```python
from build123d import *

# Parameters (mm, degrees)
BOSS_EXTRUDE1_START = -19300
BOSS_EXTRUDE1_DEPTH = 450


with BuildPart() as part:
    # Sketch1 → Boss-Extrude1 (new body)
    with BuildSketch(Plane(origin=(0, 0, 0), x_dir=(1, 0, 0), z_dir=(0, 1, 0)).offset(BOSS_EXTRUDE1_START)):
        Polygon((175, 300), (-175, 300), (-275, 200), (-200, -300), (-25, -300), (-25, -200), (25, -200), (25, -300), (200, -300), (275, 200), align=None)
    extrude(amount=BOSS_EXTRUDE1_DEPTH)


solid = part.part
```
Build history of the part. All positions in model axes, mm. A direction names the side the tool comes from. Give positions to 0.01 mm unless a question says otherwise; leave off trailing zeros. Loops run counter-clockwise (first coordinate to the right, second up) from the corner with the lowest first, then second, coordinate; pieces in that order, holes last.
1) 3-axis set-ups, long thin cutter, end or side, ignore diameter. For faces 1 (the face through (25, -19078, 249)), 2 (the face through (-4, -19300, -4)): which of +Z, -Z, +X, -X, +Y, -Y reach the whole face in a straight line?
Values follow:
face 1: +Z, +Y, -Y
face 2: +Z, -Z, +X, -X, -Y
2) Drop flat-ended pins along their axis: P1, Ø1, axis at y = -19121, z = -216, coming from the -X side; P2, Ø2, axis at y = -18961, z = -170.5, coming from the -X side (3 decimals); P3, Ø2, axis at x = 217, y = -18906, coming from the -Z side. Give the stop position or say it passes through.
Values follow:
P1: stops at x = -259.5
P2: stops at x = -270.725
P3: stops at z = -259
3) Probe line 1 along Z through (x, y) = (-14.5, -19253.5); line 2 along X through (y, z) = (-19201.5, 215); line 3 along X through (y, z) = (-19075.5, -129). List the from-to ranges inside material, lowest first.
Values follow:
line 1: z = -300 to 200
line 2: x = -212.75 to -25, 25 to 212.75
line 3: x = -264.35 to 264.35
4) Band-saw the part on A-A on y = -19175. List the corners of the cut face in (x, z), then the cut area to 4 significant figures.
Values follow:
outline: (-275, -200) - (-175, -300) - (175, -300) - (275, -200) - (200, 300) - (25, 300) - (25, 200) - (-25, 200) - (-25, 300) - (-200, 300) - close
area: 277,500 mm2
5) Band-saw the part on B-B on z = 138. List the corners of the cut face in (x, y).
Values follow:
outline: (-224.3, -19300) - (224.3, -19300) - (224.3, -18850) - (-224.3, -18850) - close
6) Two-plate mould, pull along X, no slides. Class faces 3 (the face through (226, -19078, -249)), 4 (the face through (0, -19078, 200)), 5 (the face through (2, -19078, -300)), 6 (the face through (-238.025, -19078.15, 46.5)): released by +X, released by -X, zero draft, split by the parting line, or undercut.
Values follow:
face 3: released by +X
face 4: undercut
face 5: zero draft
face 6: released by -X
7) Band-saw the part on C-C on x = -13.5. List the corners of the cut face in (y, z), then the cut area to 3 significant figures.
Values follow:
outline: (-19300, -300) - (-18850, -300) - (-18850, 200) - (-19300, 200) - close
area: 225,000 mm2
